For this review, take the finished solid that the model builds, in its own axes (mm). A direction names the side the tool comes from. Round coordinates to 2 decimals unless told otherwise and drop trailing zeros. Order: outer loops, then holes, each group sorted by start corner. A loop starts at its lowest first (then second) coordinate and runs counter-clockwise, first axis right, second up.
```python
from build123d import *

# Parameters (mm, degrees)
SKETCH2_W           = 20
SKETCH2_H           = 29.6
BOSS_EXTRUDE1_DEPTH = 4
SKETCH3_W           = 20
SKETCH3_H           = 4
BOSS_EXTRUDE2_DEPTH = 20
SKETCH4_W           = 20
SKETCH4_H           = 4
BOSS_EXTRUDE3_DEPTH = 16
SKETCH5_W           = 4
SKETCH5_H           = 20
BOSS_EXTRUDE4_DEPTH = 15
SKETCH6_W           = 4
SKETCH6_H           = 20
BOSS_EXTRUDE5_DEPTH = 15
FILLET1_R           = 5
FILLET3_R           = 0.5
CUT_EXTRUDE2_REACH  = 41.548
SKETCH9_R           = 3
CUT_EXTRUDE3_REACH  = 39.256
SKETCH10_R          = 3


with BuildPart() as part:
    # Sketch2 → Boss-Extrude1 (new body)
    with BuildSketch(Plane(origin=(0, 0, 0), x_dir=(0, 0, -1), z_dir=(1, 0, 0))):
        Rectangle(SKETCH2_W, SKETCH2_H)
    extrude(amount=BOSS_EXTRUDE1_DEPTH)

    # Sketch3 → Boss-Extrude2 (add)
    with BuildSketch(Plane(origin=(4, 0, 0), x_dir=(0, 0, -1), z_dir=(1, 0, 0))):
        with Locations((0, 12.8)):
            Rectangle(SKETCH3_W, SKETCH3_H)
    extrude(amount=BOSS_EXTRUDE2_DEPTH)

    # Sketch4 → Boss-Extrude3 (add)
    with BuildSketch(Plane(origin=(4, 0, 0), x_dir=(0, 0, -1), z_dir=(1, 0, 0))):
        with Locations((0, -12.8)):
            Rectangle(SKETCH4_W, SKETCH4_H)
    extrude(amount=BOSS_EXTRUDE3_DEPTH)

    # Sketch5 → Boss-Extrude4 (add)
    with BuildSketch(Plane(origin=(0, 14.8, 0), x_dir=(1, 0, 0), z_dir=(0, 1, 0))):
        with Locations((22, 0)):
            Rectangle(SKETCH5_W, SKETCH5_H)
    extrude(amount=BOSS_EXTRUDE4_DEPTH)

    # Sketch6 → Boss-Extrude5 (add)
    with BuildSketch(Plane.XZ.offset(14.8)):
        with Locations((18, 0)):
            Rectangle(SKETCH6_W, SKETCH6_H)
    extrude(amount=BOSS_EXTRUDE5_DEPTH)

    # Fillet1
    fillet1_edges = [part.edges().sort_by_distance(p)[0] for p in [
        (22, 29.8, -10),
        (22, 29.8, 10),
        (18, -29.8, 10),
        (18, -29.8, -10),
    ]]
    fillet(fillet1_edges, radius=FILLET1_R)

    # Fillet3
    fillet3_edges = [part.edges().sort_by_distance(p)[0] for p in [
        (4, 0, 10),
        (14, 10.8, 10),
        (14, 10.8, -10),
        (24, 10.8, 0),
        (24, 17.8, -10),
        (4, 0, -10),
        (12, -10.8, 10),
        (12, -10.8, -10),
        (20, -17.8, 10),
        (20, -10.8, 0),
        (10, 14.8, 10),
        (10, 14.8, -10),
        (20, 14.8, 0),
        (0, -14.8, 0),
        (8, -14.8, -10),
        (8, -14.8, 10),
        (16, -14.8, 0),
        (0, 0, 10),
        (0, 14.8, 0),
        (0, 0, -10),
        (20, -29.8, 0),
        (16, -29.8, 0),
        (16, -19.8, -10),
        (16, -19.8, 10),
        (16, -28.335533906, -8.535533906),
        (16, -28.335533906, 8.535533906),
        (24, 17.8, 10),
        (20, 19.8, 10),
        (20, -17.8, -10),
        (20, -28.335533906, -8.535533906),
        (20, -28.335533906, 8.535533906),
        (20, 19.8, -10),
        (24, 29.8, 0),
        (20, 29.8, 0),
        (20, 28.335533906, 8.535533906),
        (20, 28.335533906, -8.535533906),
        (24, 28.335533906, 8.535533906),
        (24, 28.335533906, -8.535533906),
    ]]
    fillet(fillet3_edges, radius=FILLET3_R)

    # Sketch9 → Cut-Extrude2 (cut, up to next)
    with BuildSketch(Plane(origin=(24, 0, 0), x_dir=(0, 0, -1), z_dir=(1, 0, 0)), mode=Mode.PRIVATE) as cut_extrude2_sk1:
        with Locations((0, 20.3)):
            Circle(SKETCH9_R)
    cut_extrude2_tool1 = extrude(cut_extrude2_sk1.sketch, amount=-CUT_EXTRUDE2_REACH, mode=Mode.PRIVATE) & part.part
    add(cut_extrude2_tool1.solids().sort_by_distance((24, 20.3, 0))[0], mode=Mode.SUBTRACT)

    # Sketch10 → Cut-Extrude3 (cut, up to next)
    with BuildSketch(Plane(origin=(20, 0, 0), x_dir=(0, 0, -1), z_dir=(1, 0, 0)), mode=Mode.PRIVATE) as cut_extrude3_sk1:
        with Locations((0, -20.3)):
            Circle(SKETCH10_R)
    cut_extrude3_tool1 = extrude(cut_extrude3_sk1.sketch, amount=-CUT_EXTRUDE3_REACH, mode=Mode.PRIVATE) & part.part
    add(cut_extrude3_tool1.solids().sort_by_distance((20, -20.3, 0))[0], mode=Mode.SUBTRACT)


solid = part.part
```
Q1. Mouldability with a two-part tool opening along Y and no side actions: class faces 5 (the face through (22.03, 22.83, -1.61)), 6 (the face through (22.02, 28.37, -8.5)), 7 (the face through (18.02, -28.37, -8.5)) as +Y half, -Y half, draft (parallel to the pull), parting line (faces both ways), or undercut.
Q2. Take a section at D-D, the plane z = 0. Count the separate pieces of the cut face and the enclosed holes in it, plus the area to 3 significant figures.
Q3. Take a section at B-B, the plane y = -20.3. State the section outline as (x, z) points.
Q4. Take a section at A-A, the plane x = 18. State the section outline as (y, z) points, plus the area to 3 significant figures.
Q5. Clearance check with flat-ended pins moving along their axes: pin 1 (6 mm diameter, centred on y = 24, z = -3, fed in from -X); pin 2 (5.5 mm diameter, centred on y = -1, z = 2.5, fed in from +X); pin 3 (6 mm diameter, centred on x = 7.5, z = 7, fed in from +Y). State where each tip first meets the part, or that it passes through.
Q6. Take a section at C-C, the plane x = 8. State the section outline as (y, z) points.
Q7. Wall thickness on line 1 (Y direction, x = 18.6, z = 0); line 2 (Y direction, x = 10.25, z = -7.5); line 3 (Y direction, x = 18.5, z = 3.75): over which ranges is each line inside the solid? List them lowest first.
Q8. Tool access review of faces 1 (the face through (8, -14.8, 0)), 2 (the face through (20, -16, 0)), 3 (the face through (4, 0, 0)), 4 (the face through (10, 14.8, 0)): name each direction out of +Z, -Z, +X, -X, +Y, -Y from which nothing blocks a thin tool from reaching the whole face with its end or side.
Working result:
1. face 5: undercut
1. face 6: +Y half
1. face 7: -Y half
2. separate pieces: 3
2. enclosed holes: 0
2. area: 334 mm2
3. outline: (16, -9.5) arc R0.5 ccw to (16.5, -10) - (19.5, -10) arc R0.5 ccw to (20, -9.5) - (20, -3) - (16, -3) - close; (16, 3) - (20, 3) - (20, 9.5) arc R0.5 ccw to (19.5, 10) - (16.5, 10) arc R0.5 ccw to (16, 9.5) - close
4. outline: (-29.8, -5) arc R5 ccw to (-24.8, -10) - (-11.3, -10) arc R0.5 ccw to (-10.8, -9.5) - (-10.8, 9.5) arc R0.5 ccw to (-11.3, 10) - (-24.8, 10) arc R5 ccw to (-29.8, 5) - close; (10.8, -9.5) arc R0.5 ccw to (11.3, -10) - (14.3, -10) arc R0.5 ccw to (14.8, -9.5) - (14.8, 9.5) arc R0.5 ccw to (14.3, 10) - (11.3, 10) arc R0.5 ccw to (10.8, 9.5) - close; hole circle Ø6 at (-20.3, 0)
4. area: 421 mm2
5. pin 1: stops at x = 20
5. pin 2: stops at x = 4
5. pin 3: stops at y = 14.8
6. outline: (-14.8, -9.5) arc R0.5 ccw to (-14.3, -10) - (-11.3, -10) arc R0.5 ccw to (-10.8, -9.5) - (-10.8, 9.5) arc R0.5 ccw to (-11.3, 10) - (-14.3, 10) arc R0.5 ccw to (-14.8, 9.5) - close; (10.8, -9.5) arc R0.5 ccw to (11.3, -10) - (14.3, -10) arc R0.5 ccw to (14.8, -9.5) - (14.8, 9.5) arc R0.5 ccw to (14.3, 10) - (11.3, 10) arc R0.5 ccw to (10.8, 9.5) - close
7. line 1: y = -29.8 to -23.3, -17.3 to -10.8, 10.8 to 14.8
7. line 2: y = -14.8 to -10.8, 10.8 to 14.8
7. line 3: y = -29.8 to -10.8, 10.8 to 14.8
8. face 1: +Z, -Z, -X, -Y
8. face 2: +Z, -Z, +X, -Y
8. face 3: +Z, -Z, +X
8. face 4: +Z, -Z, -X, +Y
